Here's how the part is built. I have some questions about the finished solid (model axes, mm). Face numbers are marked on the shaded views. A direction names the side the tool comes from. Give positions to 0.01 mm unless a question says otherwise; leave off trailing zeros. Write each loop counter-clockwise with the first axis right and the second up, starting at its lowest first coordinate (ties: lowest second). Pieces come first, ordered by that corner, then holes. Notation, with made-up numbers: (71, 46.25) -> (122, 46.25) arc R24 cw to (122, 64.25) -> close; hole circle Ø10 at (-34.5, 89). An arc over 180 degrees is marked (long way). Use CSV: the item, a comma, the result in double quotes. Start each with the question number.
(1) For pin 1 Ø2.5 at (x, y) = (36, 5) entering from -Z; pin 2 Ø4.5 at (x, y) = (6, 11.5) entering from +Z; pin 3 Ø1.2 at (x, y) = (39, 5) entering from +Z, each with a flat end and sliding along its axis, tell me the tip position at first contact or that it passes through.
(2) Suppose I cut it at C-C on y = 9.25. List the corners of the cut face in (x, z) for me.
(3) If we mould it in two halves opening along X, with no side actions, what happens to the marked faces 1, 2 and 3? For each: pulls with the +X half, pulls with the -X half, needs draft (parallel to the pull), parting line crosses it, or undercut.
(4) Suppose I cut it at D-D on x = 15.5. List the corners of the cut face in (y, z) for me, plus the area to 3 significant figures.
(5) I need wall thicknesses on L1, parallel to Y at x = 33, z = -0.45; L2, parallel to X at y = 17.75, z = -1; L3, parallel to Y at x = 41.65, z = 0. Which ranges of each line are inside material? Lowest first, please. Write a range as [from, to].
(6) Suppose I cut it at B-B on x = 20. List the corners of the cut face in (y, z) for me.
(7) Which directions (+Z, -Z, +X, -X, +Y, -Y) give clear straight access to the entire face, cutting with the end or side of a thin tool? Please do the marked faces 4 and 5.
(8) Suppose I cut it at A-A on z = 0. Give the number of separate pieces and of enclosed holes in the cut face, plus the area to 3 significant figures.
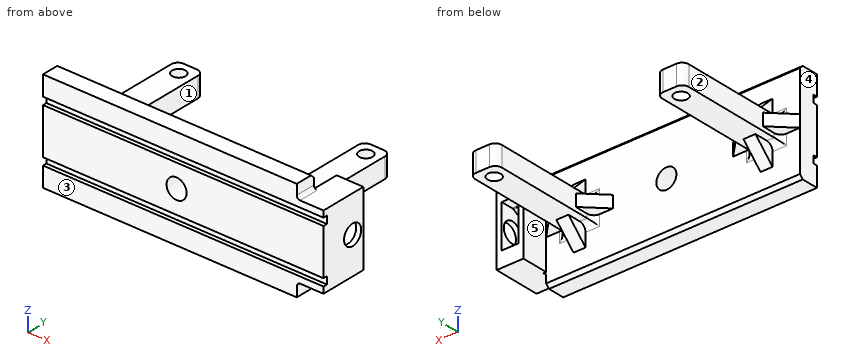
from build123d import *

# Parameters (mm, degrees)
CROQUIS1_R                   = 1
SALIENTE_EXTRUIR1_DEPTH      = 1.5
CROQUIS2_W                   = 38
CROQUIS2_H                   = 3
SALIENTE_EXTRUIR2_DEPTH      = 6
CROQUIS3_W                   = 38
CROQUIS3_H                   = 3
SALIENTE_EXTRUIR3_DEPTH      = 6
REDONDEO1_R                  = 1
NERVIO1_REACH                = 45.592
CROQUIS4_WALL_W              = 93.426354762
CROQUIS4_WALL_H              = 1.8
NERVIO5_REACH                = 45.592
CROQUIS5_WALL_W              = 93.426354762
CROQUIS5_WALL_H              = 1.8
NERVIO6_REACH                = 41.31
CROQUIS6_WALL_W              = 84.861976732
CROQUIS6_WALL_H              = 1.8
NERVIO7_REACH                = 41.31
CROQUIS7_WALL_W              = 84.861976732
CROQUIS7_WALL_H              = 1.8
REDONDEO2_R                  = 1
CROQUIS8_W                   = 38
CROQUIS8_H                   = 1.1
CROQUIS8_W_2                 = 38.249115133
CORTAR_EXTRUIR1_DEPTH        = 0.6
SALIENTE_EXTRUIR5_DEPTH      = 4
SALIENTE_EXTRUIR5_DEPTH_BACK = 3
CROQUIS10_W                  = 4
CROQUIS10_H                  = 11
CORTAR_EXTRUIR2_START        = -2
CORTAR_EXTRUIR2_DEPTH        = 1.25
REDONDEO5_R                  = 0.5
CROQUIS13_W                  = 4
CROQUIS13_H                  = 1.1
CORTAR_EXTRUIR4_DEPTH        = 0.6
CROQUIS14_W                  = 2.5
CROQUIS14_H                  = 6.410956056
CORTAR_EXTRUIR5_DEPTH        = 2
CORTAR_EXTRUIR6_START        = -3.25
CROQUIS11_3_R                = 1.5
CORTAR_EXTRUIR6_DEPTH        = 4
CORTAR_EXTRUIR7_REACH        = 47.927
CROQUIS16_R                  = 1.5
REDONDEO6_R                  = 0.5
CHAFL_N1_SIZE                = 0.5


with BuildPart() as part:
    # Croquis1 → Saliente-Extruir1 (new, symmetric)
    with BuildSketch(Plane.XY):
        Polygon((0, 0), (38, 0), (38, 3), (35, 3), (35, 20), (31, 20), (31, 3), (7, 3), (7, 20), (3, 20), (3, 3), (0, 3), align=None)
        with Locations((5, 18)):
            Circle(CROQUIS1_R, mode=Mode.SUBTRACT)
        with Locations((33, 18)):
            Circle(CROQUIS1_R, mode=Mode.SUBTRACT)
    extrude(amount=SALIENTE_EXTRUIR1_DEPTH, both=True)

    # Croquis2 → Saliente-Extruir2 (add)
    with BuildSketch(Plane.XY.offset(1.5)):
        with Locations((19, 1.5)):
            Rectangle(CROQUIS2_W, CROQUIS2_H)
    extrude(amount=SALIENTE_EXTRUIR2_DEPTH)

    # Croquis3 → Saliente-Extruir3 (add)
    with BuildSketch(Plane(origin=(0, 0, -1.5), x_dir=(-1, 0, 0), z_dir=(0, 0, -1))):
        with Locations((-19, 1.5)):
            Rectangle(CROQUIS3_W, CROQUIS3_H)
    extrude(amount=SALIENTE_EXTRUIR3_DEPTH)

    # Redondeo1
    redondeo1_edges = [part.edges().sort_by_distance(p)[0] for p in [
        (3, 20, 0),
        (7, 20, 0),
        (31, 20, 0),
        (35, 20, 0),
    ]]
    fillet(redondeo1_edges, radius=REDONDEO1_R)

    # Croquis4 wall → Nervio1 (add, up to next)
    with BuildSketch(Plane(origin=(36.5, 4.5, 0), x_dir=(0.707106781187, -0.707106781187, 0), z_dir=(0.707106781187, 0.707106781187, 0)), mode=Mode.PRIVATE) as nervio1_sk1:
        Rectangle(CROQUIS4_WALL_W, CROQUIS4_WALL_H)
    nervio1_tool1 = extrude(nervio1_sk1.sketch, amount=-NERVIO1_REACH, mode=Mode.PRIVATE) - part.part
    nervio1 = nervio1_tool1.solids().sort_by_distance((36.5, 4.5, 0))[0]
    add(nervio1)

    # Croquis5 wall → Nervio5 (add, up to next)
    with BuildSketch(Plane(origin=(29.5, 4.5, 0), x_dir=(-0.707106781187, -0.707106781187, 0), z_dir=(0.707106781187, -0.707106781187, 0)), mode=Mode.PRIVATE) as nervio5_sk1:
        Rectangle(CROQUIS5_WALL_W, CROQUIS5_WALL_H)
    nervio5_tool1 = extrude(nervio5_sk1.sketch, amount=NERVIO5_REACH, mode=Mode.PRIVATE) - part.part
    nervio5 = nervio5_tool1.solids().sort_by_distance((29.5, 4.5, 0))[0]
    add(nervio5)

    # Croquis6 wall → Nervio6 (add, up to next)
    with BuildSketch(Plane(origin=(33, 4.5, -3), x_dir=(0, -0.707106781187, -0.707106781187), z_dir=(0, 0.707106781187, -0.707106781187)), mode=Mode.PRIVATE) as nervio6_sk1:
        Rectangle(CROQUIS6_WALL_W, CROQUIS6_WALL_H)
    nervio6_tool1 = extrude(nervio6_sk1.sketch, amount=-NERVIO6_REACH, mode=Mode.PRIVATE) - part.part
    nervio6 = nervio6_tool1.solids().sort_by_distance((33, 4.5, -3))[0]
    add(nervio6)

    # Croquis7 wall → Nervio7 (add, up to next)
    with BuildSketch(Plane(origin=(33, 4.5, 3), x_dir=(0, -0.707106781187, 0.707106781187), z_dir=(0, -0.707106781187, -0.707106781187)), mode=Mode.PRIVATE) as nervio7_sk1:
        Rectangle(CROQUIS7_WALL_W, CROQUIS7_WALL_H)
    nervio7_tool1 = extrude(nervio7_sk1.sketch, amount=NERVIO7_REACH, mode=Mode.PRIVATE) - part.part
    nervio7 = nervio7_tool1.solids().sort_by_distance((33, 4.5, 3))[0]
    add(nervio7)

    # Simetría3: Nervio1, Nervio5, Nervio6, Nervio7 across plane
    add(nervio1.mirror(Plane.ZY.offset(-19)))
    add(nervio5.mirror(Plane.ZY.offset(-19)))
    add(nervio6.mirror(Plane.ZY.offset(-19)))
    add(nervio7.mirror(Plane.ZY.offset(-19)))

    # Redondeo2
    redondeo2_edges = [part.edges().sort_by_distance(p)[0] for p in [
        (35, 3, -1.2),
        (31, 3, -1.2),
        (34.45, 3, -1.5),
        (3, 3, 1.2),
        (7, 3, 1.2),
        (31.55, 3, 1.5),
        (31, 3, 1.2),
        (35, 3, 1.2),
        (3, 3, -1.2),
        (7, 3, -1.2),
        (6.45, 3, -1.5),
        (3.55, 3, 1.5),
        (6.45, 3, 1.5),
        (34.45, 3, 1.5),
        (31.55, 3, -1.5),
        (3.55, 3, -1.5),
    ]]
    fillet(redondeo2_edges, radius=REDONDEO2_R)

    # Croquis8 → Cortar-Extruir1 (cut)
    with BuildSketch(Plane.XZ):
        with Locations((19, 4)):
            Rectangle(CROQUIS8_W, CROQUIS8_H)
        with Locations((19.124557567, -4)):
            Rectangle(CROQUIS8_W_2, CROQUIS8_H)
    extrude(amount=-CORTAR_EXTRUIR1_DEPTH, mode=Mode.SUBTRACT)

    # Croquis10 → Saliente-Extruir5 (add, two sides: drawn at the far end of the back side and taken through both)
    with BuildSketch(Plane(origin=(0, 3, 0), x_dir=(1, 0, 0), z_dir=(0, 1, 0)).offset(-SALIENTE_EXTRUIR5_DEPTH_BACK)):
        with Locations((40, 0)):
            Rectangle(CROQUIS10_W, CROQUIS10_H)
    extrude(amount=SALIENTE_EXTRUIR5_DEPTH + SALIENTE_EXTRUIR5_DEPTH_BACK)

    # Croquis11 → Cortar-Extruir2 (cut, symmetric)
    with BuildSketch(Plane.ZY.offset(-38).offset(CORTAR_EXTRUIR2_START)):
        Polygon((1.645448267, 2.27), (3.290896534, 5.12), (1.645448267, 7.97), (-1.645448267, 7.97), (-3.290896534, 5.12), (-1.645448267, 2.27), align=None)
    extrude(amount=CORTAR_EXTRUIR2_DEPTH, both=True, mode=Mode.SUBTRACT)

    # Redondeo5
    redondeo5_edges = [part.edges().sort_by_distance(p)[0] for p in [
        (40, 5.12, -3.290896534),
        (40, 2.27, -1.645448267),
        (40, 2.27, 1.645448267),
        (40, 5.12, 3.290896534),
    ]]
    fillet(redondeo5_edges, radius=REDONDEO5_R)

    # Croquis13 → Cortar-Extruir4 (cut)
    with BuildSketch(Plane.XZ):
        with Locations((40, 4)):
            Rectangle(CROQUIS13_W, CROQUIS13_H)
        with Locations((40, -4)):
            Rectangle(CROQUIS13_W, CROQUIS13_H)
    extrude(amount=-CORTAR_EXTRUIR4_DEPTH, mode=Mode.SUBTRACT)

    # Croquis14 → Cortar-Extruir5 (cut)
    with BuildSketch(Plane(origin=(0, 7, 0), x_dir=(1, 0, 0), z_dir=(0, 1, 0))):
        with Locations((40, 0)):
            Rectangle(CROQUIS14_W, CROQUIS14_H)
    extrude(amount=-CORTAR_EXTRUIR5_DEPTH, mode=Mode.SUBTRACT)

    # Croquis11<3> → Cortar-Extruir6 (cut)
    with BuildSketch(Plane.ZY.offset(-38).offset(CORTAR_EXTRUIR6_START)):
        with Locations((0, 5.12)):
            Circle(CROQUIS11_3_R)
    extrude(amount=-CORTAR_EXTRUIR6_DEPTH, mode=Mode.SUBTRACT)

    # Croquis16 → Cortar-Extruir7 (cut, up to next)
    with BuildSketch(Plane(origin=(0, 3, 0), x_dir=(1, 0, 0), z_dir=(0, 1, 0)), mode=Mode.PRIVATE) as cortar_extruir7_sk1:
        with Locations(Location((20, 0, 0), (0, 0, 270))):
            Circle(CROQUIS16_R)
    cortar_extruir7_tool1 = extrude(cortar_extruir7_sk1.sketch, amount=-CORTAR_EXTRUIR7_REACH, mode=Mode.PRIVATE) & part.part
    add(cortar_extruir7_tool1.solids().sort_by_distance((20, 3, 0))[0], mode=Mode.SUBTRACT)

    # Redondeo6
    redondeo6_edges = [part.edges().sort_by_distance(p)[0] for p in [
        (38, 1.5, 5.5),
        (38, 1.5, -5.5),
    ]]
    fillet(redondeo6_edges, radius=REDONDEO6_R)

    # Chaflán1
    chafl_n1_edges = [part.edges().sort_by_distance(p)[0] for p in [
        (19, 3, 7.5),
        (19, 3, -7.5),
    ]]
    chamfer(chafl_n1_edges, length=CHAFL_N1_SIZE)


solid = part.part
Geometry says:
1,pin 1,"z = -1.5"
1,pin 2,"z = 1.5"
1,pin 3,"z = 5.5"
2,outline,"(3, -1.5) -> (7, -1.5) -> (7, 1.5) -> (3, 1.5) -> close; (31, -1.5) -> (35, -1.5) -> (35, 1.5) -> (31, 1.5) -> close"
3,face 1,"undercut"
3,face 2,"pulls with the -X half"
3,face 3,"needs draft"
4,outline,"(0, -7.5) -> (2.5, -7.5) -> (3, -7) -> (3, 7) -> (2.5, 7.5) -> (0, 7.5) -> (0, 4.55) -> (0.6, 4.55) -> (0.6, 3.45) -> (0, 3.45) -> (0, -3.45) -> (0.6, -3.45) -> (0.6, -4.55) -> (0, -4.55) -> close"
4,area,"43.4 mm²"
5,L1,"[0, 17], [19, 20]"
5,L2,"[3, 4.03], [5.97, 7], [31, 32.03], [33.97, 35]"
5,L3,"[0, 3.62], [6.62, 7]"
6,outline,"(0, -7.5) -> (2.5, -7.5) -> (3, -7) -> (3, -1.5) -> (0, -1.5) -> (0, -3.45) -> (0.6, -3.45) -> (0.6, -4.55) -> (0, -4.55) -> close; (0, 1.5) -> (3, 1.5) -> (3, 7) -> (2.5, 7.5) -> (0, 7.5) -> (0, 4.55) -> (0.6, 4.55) -> (0.6, 3.45) -> (0, 3.45) -> close"
7,face 4,"+Z, -Z, -X, +Y, -Y"
7,face 5,"+Z, -Z, +Y"
8,separate pieces,"3"
8,enclosed holes,"2"
8,area,"266 mm²"
